The listing builds one solid part. Answer for the finished solid, in the listing's coordinates (mm). A direction names the side the tool comes from. Give positions to 0.01 mm unless a question says otherwise; leave off trailing zeros. Order: outer loops, then holes, each group sorted by start corner. A loop starts at its lowest first (then second) coordinate and runs counter-clockwise, first axis right, second up. Notation, with made-up numbers: (32.25, 3) -> (66.25, 3) arc R36 cw to (66.25, 39) -> close; hole circle Ø5 at (42.5, 40). An arc over 180 degrees is marked (long way). Write item = value, one per line. Start each with the question number.
```python
from build123d import *

# Parameters (mm, degrees)
F0_W     = 101.6
F0_H     = 50.8
F1_DEPTH = 127
F2_T     = -3.175
F4_D     = 7.9375
F4_DEPTH = 12.7
F5_W     = 21.021394
F5_H     = 7.722143
F6_DEPTH = 3.175


with BuildPart() as f1:
    # F0 (on Front) → F1 (new body)
    with BuildSketch(Plane.XZ):
        with Locations((-34.801298, 25.4)):
            Rectangle(F0_W, F0_H)
    extrude(amount=F1_DEPTH)

    # F2
    f2_openings = [f1.faces().sort_by_distance(p)[0] for p in [
        (-34.801298, -63.5, 50.8),
    ]]
    offset(amount=F2_T, openings=f2_openings)

    # F4
    with Locations(Plane.XZ.offset(127)):
        with Locations((-62.723987, 27.134759)):
            Hole(F4_D / 2, depth=F4_DEPTH)

    # F5 (on face) → F6 (cut, through all)
    with BuildSketch(Plane.XZ.offset(127)):
        with Locations((-24.327768, 29.708806)):
            Rectangle(F5_W, F5_H)
    extrude(amount=-F6_DEPTH, mode=Mode.SUBTRACT)


solid = f1.part
```
Item 1: Which of the six approach directions +Z, -Z, +X, -X, +Y, -Y give full straight-line access (tool end or side, diameter ignored) to faces 1 (the flat face through (-82.426, -63, 27)), 2 (the flat face through (-24, -125, 33.57)), 3 (the flat face through (-36, -63, 0))?
Item 2: Flat-ended cylindrical pins translate along their axes: pin 1 (8 mm diameter, centred on x = -53, z = 37, fed in from +Y); pin 2 (4 mm diameter, centred on x = -61, z = 27.5, fed in from -Y) (3 decimals); pin 3 (3 mm diameter, centred on x = -46, y = -112, fed in from +Z) (3 decimals). Find the tip coordinate at first contact, or state that the pin passes through.
Item 3: A cutting plane is placed at A-A, the plane x = -23. Write down the section's boundary in (y, z) (3 decimals), plus the area to 3 significant figures.
Item 4: Consider L1, parallel to X at y = -31, z = 36; L2, parallel to Y at x = -57, z = 21 (3 decimals); L3, parallel to Z at x = -20, y = -84 (3 decimals). Determine where each line is inside the solid, lowest interval first. Write a range as from..to.
Item 5: A cutting plane is placed at D-D, the plane z = 29. Write down the section's boundary in (x, y) (3 decimals), plus the area to 3 significant figures.
Item 6: The mould has two halves that part along Z. Classify faces 4 (the flat face through (-35, -63, 3.175)), 5 (the cylindrical face through (-58.76, -125.39, 27.31)), 6 (the flat face through (15.999, -63, 25)), 7 (the flat face through (-13.817, -125, 30)): +Z half, -Z half, draft (parallel to the pull), parting line (faces both ways), or undercut.
Item 7: A cutting plane is placed at B-B, the plane z = 19.5. Write down the section's boundary in (x, y) (3 decimals), plus the area to 3 significant figures.
Item 8: A cutting plane is placed at C-C, the plane y = -34. Write down the section's boundary in (x, z) (3 decimals).
Check values:
q1.face_1 = +Z
q1.face_2 = -Y
q1.face_3 = -Z, +X, -X, +Y, -Y
q2.pin_1 = 0
q2.pin_2 = -3.175
q2.pin_3 = 3.175
q3.outline = (-127, 0) -> (0, 0) -> (0, 50.8) -> (-3.175, 50.8) -> (-3.175, 3.175) -> (-123.825, 3.175) -> (-123.825, 25.848) -> (-127, 25.848) -> close; (-127, 33.57) -> (-123.825, 33.57) -> (-123.825, 50.8) -> (-127, 50.8) -> close
q3.area = 681 mm^2
q4.L1 = -85.6..-82.43, 12.82..16
q4.L2 = -127..-123.825, -3.175..0
q4.L3 = 0..3.175
q5.outline = (-85.601, -127) -> (-66.227, -127) -> (-66.227, -123.825) -> (-82.426, -123.825) -> (-82.426, -3.175) -> (12.824, -3.175) -> (12.824, -123.825) -> (-13.817, -123.825) -> (-13.817, -127) -> (15.999, -127) -> (15.999, 0) -> (-85.601, 0) -> close; (-59.221, -127) -> (-34.838, -127) -> (-34.838, -123.825) -> (-59.221, -123.825) -> close
q5.area = 1,320 mm^2
q6.face_4 = +Z half
q6.face_5 = undercut
q6.face_6 = draft
q6.face_7 = undercut
q7.outline = (-85.601, -127) -> (15.999, -127) -> (15.999, 0) -> (-85.601, 0) -> close; hole (-82.426, -123.825) -> (12.824, -123.825) -> (12.824, -3.175) -> (-82.426, -3.175) -> close
q7.area = 1,410 mm^2
q8.outline = (-85.601, 0) -> (15.999, 0) -> (15.999, 50.8) -> (12.824, 50.8) -> (12.824, 3.175) -> (-82.426, 3.175) -> (-82.426, 50.8) -> (-85.601, 50.8) -> close
